from build123d import *

# Parameters (mm, degrees)
F0_W      = 20
F0_H      = 20
F1_DEPTH  = 20
F2_R      = 1.5
F3_DEPTH  = 2
F4_R      = 1.5
F5_DEPTH  = 2
F6_R      = 1.5
F7_DEPTH  = 2
F8_R      = 1.5
F9_DEPTH  = 2
F10_R     = 1.5
F11_DEPTH = 2
F12_R     = 1.5
F13_DEPTH = 2


with BuildPart() as f1:
    # F0 (on Top) → F1 (new body)
    with BuildSketch(Plane.XY):
        with Locations((-22.53249, -11.250252)):
            Rectangle(F0_W, F0_H)
    extrude(amount=F1_DEPTH)

    # F2 (on face) → F3 (cut)
    with BuildSketch(Plane.XY.offset(20)):
        with Locations((-22.833129, -11.315533)):
            Circle(F2_R)
    extrude(amount=-F3_DEPTH, mode=Mode.SUBTRACT)

    # F4 (on face) → F5 (cut)
    with BuildSketch(Plane.XZ.offset(21.250252)):
        with Locations((-28.556654, 15.928326)):
            Circle(F4_R)
        with Locations((-16.452408, 4.484393)):
            Circle(F4_R)
    extrude(amount=-F5_DEPTH, mode=Mode.SUBTRACT)

    # F6 (on face) → F7 (cut)
    with BuildSketch(Plane.YZ.offset(-12.53249)):
        with Locations((-11.837029, 16.616692)):
            Circle(F6_R)
        with Locations((-11.448925, 3.613711)):
            Circle(F6_R)
        with Locations((-11.627831, 10.102251)):
            Circle(F6_R)
    extrude(amount=-F7_DEPTH, mode=Mode.SUBTRACT)

    # F8 (on face) → F9 (cut)
    with BuildSketch(Plane(origin=(0, -1.250252, 0), x_dir=(-1, 0, 0), z_dir=(0, 1, 0))):
        with Locations((16.232165, 16.211085)):
            Circle(F8_R)
        with Locations((29.102561, 16.407891)):
            Circle(F8_R)
        with Locations((28.863132, 3.995854)):
            Circle(F8_R)
        with Locations((16.077781, 4.228219)):
            Circle(F8_R)
    extrude(amount=-F9_DEPTH, mode=Mode.SUBTRACT)

    # F10 (on face) → F11 (cut)
    with BuildSketch(Plane(origin=(-32.53249, 0, 0), x_dir=(0, -1, 0), z_dir=(-1, 0, 0))):
        with Locations((18.142659, 16.85593)):
            Circle(F10_R)
        with Locations((17.976478, 3.165177)):
            Circle(F10_R)
        with Locations((4.45046, 16.641465)):
            Circle(F10_R)
        with Locations((10.722963, 9.346528)):
            Circle(F10_R)
        with Locations((4.027196, 2.76337)):
            Circle(F10_R)
    extrude(amount=-F11_DEPTH, mode=Mode.SUBTRACT)

    # F12 (on face) → F13 (cut)
    with BuildSketch(Plane(origin=(0, 0, 0), x_dir=(1, 0, 0), z_dir=(0, 0, -1))):
        with Locations((-15.62013, 17.110417)):
            Circle(F12_R)
        with Locations((-22.286659, 17.470592)):
            Circle(F12_R)
        with Locations((-29.12412, 17.320384)):
            Circle(F12_R)
        with Locations((-29.280099, 6.113375)):
            Circle(F12_R)
        with Locations((-22.681733, 6.085219)):
            Circle(F12_R)
        with Locations((-15.74056, 5.76421)):
            Circle(F12_R)
    extrude(amount=-F13_DEPTH, mode=Mode.SUBTRACT)


solid = f1.part
Read the model definition and answer for the solid it produces. Units are mm, in the model's axes. A direction names the side the tool comes from. Coordinates: 2 decimals unless noted, no trailing zeros. Order: outer loops, then holes, each group sorted by start corner. A loop starts at its lowest first (then second) coordinate and runs counter-clockwise, first axis right, second up. Notation, with made-up numbers: (87.25, 37) -> (132.25, 37) arc R24 ccw to (132.25, 76) -> close; hole circle Ø3 at (-1.75, 71). An arc over 180 degrees is marked (long way). Answer as a JSON object with one key per item and string values.
1) A cutting plane is placed at D-D, the plane x = -28.5. Determine the outline of the cut face in (y, z).
Model answer:
{"outline": "(-21.25, 0) -> (-18.68, 0) -> (-18.68, 2) -> (-15.96, 2) -> (-15.96, 0) -> (-7.39, 0) -> (-7.39, 2) -> (-4.83, 2) -> (-4.83, 0) -> (-1.25, 0) -> (-1.25, 2.54) -> (-3.25, 2.54) -> (-3.25, 5.45) -> (-1.25, 5.45) -> (-1.25, 15.03) -> (-3.25, 15.03) -> (-3.25, 17.78) -> (-1.25, 17.78) -> (-1.25, 20) -> (-21.25, 20) -> (-21.25, 17.43) -> (-19.25, 17.43) -> (-19.25, 14.43) -> (-21.25, 14.43) -> close"}
2) A cutting plane is placed at B-B, the plane y = -6.5. Determine the outline of the cut face in (x, z), plus the area to 3 significant figures.
Model answer:
{"outline": "(-32.53, 0) -> (-30.73, 0) -> (-30.73, 2) -> (-27.83, 2) -> (-27.83, 0) -> (-24.12, 0) -> (-24.12, 2) -> (-21.24, 2) -> (-21.24, 0) -> (-17.05, 0) -> (-17.05, 2) -> (-14.43, 2) -> (-14.43, 0) -> (-12.53, 0) -> (-12.53, 20) -> (-32.53, 20) -> close", "area": "383 mm²"}
3) The mould has two halves that part along X. Classify faces 1 (the face through (-30.78, -6.18, 0.99)), 2 (the face through (-31.5, -2.8, 1.9)), 3 (the face through (-14.532, -12, 17)), 4 (the face through (-30.532, -18, 3)): released by +X, released by -X, zero draft, split by the parting line, or undercut.
Model answer:
{"face 1": "undercut", "face 2": "zero draft", "face 3": "released by +X", "face 4": "released by -X"}
4) A cutting plane is placed at C-C, the plane x = -23.25. Determine the outline of the cut face in (y, z), plus the area to 3 significant figures.
Model answer:
{"outline": "(-21.25, 0) -> (-18.62, 0) -> (-18.62, 2) -> (-16.32, 2) -> (-16.32, 0) -> (-7.47, 0) -> (-7.47, 2) -> (-4.7, 2) -> (-4.7, 0) -> (-1.25, 0) -> (-1.25, 20) -> (-9.87, 20) -> (-9.87, 18) -> (-12.76, 18) -> (-12.76, 20) -> (-21.25, 20) -> close", "area": "384 mm²"}
5) Each of these flat-tipped pins is pushed along its axis until it touches: pin 1 (0.9 mm diameter, centred on x = -29, z = 4, fed in from +Y); pin 2 (1.5 mm diameter, centred on y = -17.5, z = 17, fed in from -X). Where does it stop, or does it pass through?
Model answer:
{"pin 1": "stops at y = -3.25", "pin 2": "stops at x = -30.53"}
6) A tool of negligible diameter and unlimited length cuts with its end or side. For faces 5 (the face through (-21.402, -10.865, 19.014)), 6 (the face through (-29, -19.25, 16)), 7 (the face through (-29, -3.25, 4)), 8 (the face through (-31.546, -16.478, 3.231)), 9 (the face through (-29, -17, 2)), from which of +Z, -Z, +X, -X, +Y, -Y can it reach the whole face along a straight path? Write none if from no direction.
Model answer:
{"face 5": "+Z", "face 6": "-Y", "face 7": "+Y", "face 8": "-X", "face 9": "-Z"}
7) Consider line 1 along Z through (x, y) = (-28, -2.5); line 2 along Z through (x, y) = (-28.5, -1.75); line 3 along Y through (x, z) = (-17.5, 4.25). Determine where each line is inside the solid, lowest interval first. Write a range as from..to.
Model answer:
{"line 1": "z = 0..2.77, 5.22..15.39, 17.42..20", "line 2": "z = 0..2.54, 5.45..15.03, 17.78..20", "line 3": "y = -19.25..-3.25"}
8) A cutting plane is placed at A-A, the plane x = -15.5. Determine the outline of the cut face in (y, z), plus the area to 3 significant figures.
Model answer:
{"outline": "(-21.25, 0) -> (-18.61, 0) -> (-18.61, 2) -> (-15.62, 2) -> (-15.62, 0) -> (-7.24, 0) -> (-7.24, 2) -> (-4.28, 2) -> (-4.28, 0) -> (-1.25, 0) -> (-1.25, 2.84) -> (-3.25, 2.84) -> (-3.25, 5.61) -> (-1.25, 5.61) -> (-1.25, 14.9) -> (-3.25, 14.9) -> (-3.25, 17.52) -> (-1.25, 17.52) -> (-1.25, 20) -> (-21.25, 20) -> (-21.25, 5.64) -> (-19.25, 5.64) -> (-19.25, 3.33) -> (-21.25, 3.33) -> close", "area": "373 mm²"}
